Autodesk Inventor part; units mm, degrees
ref_plane "YZ Plane" through (0, 0, 0) normal (1, 0, 0) x (0, 1, 0)
ref_plane "XZ Plane" through (0, 0, 0) normal (0, 1, 0) x (-1, 0, 0)
ref_plane "XY Plane" through (0, 0, 0) normal (0, 0, 1) x (1, 0, 0)
sketch "Sketch1" plane through (0, 0, 0) normal (0, 1, 0) x (-1, 0, 0)
  line L0 (0, 0) -> (14, 0)
  line L1 (14, 0) -> (14, -8.75)
  line L2 (14, -8.75) -> (0, -8.75)
  line L3 (0, -8.75) -> (0, 0)
  line L4 (14, 0) -> (0, 0)
  line L5 (0, 0) -> (0, -8)
  line L6 (0, -8) -> (14, -8)
  line L7 (14, -8) -> (14, 0)
  line L8 (0, -8.75) -> (5.5, -8.75)
  line L9 (14, -8.75) -> (8.5, -8.75)
  line L10 (8.5, -8.75) -> (8.5, -4)
  line L11 (5.5, -8.75) -> (5.5, -4)
  line L12 (5.5, -8) -> (7, -8)
  line L13 (5.5, -8) -> (6.25, -8)
  line L14 (8.5, -8) -> (7, -8)
  line L15 (8.5, -8) -> (7.75, -8)
  line L16 (7.75, -8) -> (8.5, -8.75)
  line L17 (6.25, -8) -> (5.5, -8.75)
  dimension "d0" = 14
  dimension "d1" = 8.75
  dimension "d2" = 8
  dimension "d3" = 5.5
  dimension "d4" = 5.5
revolve "Revolution1" add sketch "Sketch1" angle 360 about axis through (0, 0, 0) along (-1, 0, 0) contours L0 L1 L6 L3 | L6 L11 L2 L3 | L1 L2 L10 L6 | L6 L17 L11 | L10 L16 L6
sketch "Sketch2" plane through (0, 0, 0) normal (1, 0, 0) x (0, 0, -1)
  circle A0 centre (0, 0) radius 1.5
  line L0 (-1.5, 0) -> (-1, 0)
  line L1 (-1, 0) -> (-1, 1.118)
  line L2 (-1, 0) -> (-1, -1.118)
  circle A1 centre (0, 0) radius 2.75
  dimension "d6" = 3
  dimension "d7" = 0.5
  dimension "d8" = 5.5
extrude "Extrusion1" cut sketch "Sketch2" against normal blind 10 contours A0 L2 L1
extrude "Extrusion2" cut sketch "Sketch2" against normal blind 0.6 contours L1 L0 A0 | A0 L0 L2 | A1
fillet "Fillet1" radius 20 1 edges at (0, 0, 2.75)
sketch "Sketch3" plane through (-14, 0, 0) normal (-1, 0, 0) x (0, 0, 1)
  circle A0 centre (0, 0) radius 8.75
  line L0 (0, -8.75) -> (0, -6.75)
  line L1 (0, 8.75) -> (0, 6.75)
  circle A1 centre (0, 0) radius 6.75
  dimension "d14" = 2
  dimension "d15" = 2
extrude "Extrusion3" cut sketch "Sketch3" against normal blind 1 contours A1
fillet "Fillet2" radius 0.5 1 edges at (-14, 0, -6.75)
sketch "Sketch4" plane through (-0.6, 0, 0) normal (1, 0, 0) x (0, 0, -1)
  circle A0 centre (0, 0) radius 2.75
  line L0 (-1, 1.118) -> (-1, -1.118)
  arc A1 (-1, -1.118) -> (-1, 1.118) centre (0, 0) ccw
  line L1 (1.5, 0) -> (1.6492, 0)
  line L2 (1.5, 0) -> (1.75, 0)
  circle A2 centre (0, 0) radius 1.75
  line L3 (-1, 1.118) -> (-1, -1.118)
  line L4 (-1, 0) -> (-1.25, 0)
  line L5 (-1.25, 0) -> (-1.25, 1.2247)
  line L6 (-1.25, 0) -> (-1.25, -1.2247)
  dimension "d19" = 0.25
  dimension "d20" = 0.25
extrude "Extrusion4" cut sketch "Sketch4" against normal blind 9.4 contours L0 L4 L5 A2 L2 L1 A1 | L0 A1 L1 L2 A2 L6 L4
sketch "Sketch5" plane through (-14, 0, 0) normal (-1, 0, 0) x (0, 0, 1)
  circle A0 centre (0, 0) radius 8.75
  circle A1 centre (0, 0) radius 7.25
  circle A2 centre (0, 0) radius 8.75
extrude "Extrusion5" add sketch "Sketch5" against normal blind 1 contours A0 | A1
sketch "Sketch6" plane through (-0.6, 0, 0) normal (1, 0, 0) x (0, 0, -1)
  arc A0 (-1.25, -1.2247) -> (-1.25, 1.2247) centre (0, 0) ccw
  line L0 (-1.25, -1.2247) -> (-1.25, 1.2247)
  circle A1 centre (0, 0) radius 2.75
  circle A2 centre (0, 0) radius 1.75
  line L1 (-1.25, -1.2247) -> (-1.25, 1.2247)
  line L2 (-1.25, 0) -> (-1, 0)
  line L3 (-1, 0) -> (-1, -1.4361)
  arc A3 (-1.25, -1.2247) -> (-1.25, 1.2247) centre (0, 0) ccw
  line L4 (-1, 0) -> (-1, 1.4361)
  dimension "d25" = 0.25
extrude "Extrusion6" add sketch "Sketch6" against normal blind 10 contours L0 L2 L3 A0 | L0 A0 L4 L2
properties part number "koło"
Could you check a few things on this model? Use its own coordinates, in mm. A direction names the side the tool comes from. Round coordinates to 2 decimals unless told otherwise and drop trailing zeros. Write each loop counter-clockwise with the first axis right and the second up, starting at its lowest first coordinate (ties: lowest second). Pieces come first, ordered by that corner, then holes. Notation, with made-up numbers: (-32, 40.25) - (26, 40.25) arc R16 ccw to (26, 50.25) - close; hole circle Ø7 at (51.5, 8.25). An arc over 180 degrees is marked (long way). Put each result on its own line as item: value. Start each with the question number.
(1) I want a section at A-A, the plane x = -10.5. Please give me the cut outline in (y, z).
(2) For faces 1 (the flat face through (-5, 0, 1)), 2 (the cylindrical face through (-2.712, -5.324, 6.944)), which set-ups out of +Z, -Z, +X, -X, +Y, -Y let a thin tool reach every point of the face, with its end or its side?
(3) Will these pins go through, and if not, where does the flat tip stop? pin 1 (6 mm diameter, centred on x = -6.5, z = -6, fed in from +Y) (3 decimals); pin 2 (1 mm diameter, centred on x = -2, y = 5, fed in from -Z); pin 3 (3 mm diameter, centred on y = 0, z = 0, fed in from +X).
(4) I need wall thicknesses on probe 1 along Y at (x, z) = (-7.25, 0); probe 2 along Y at (x, z) = (-4.5, 0); probe 3 along X at (y, z) = (6.5, -4.75). Which ranges of each line are inside material? Lowest first, please.
(5) I want a section at B-B, the plane x = -3. Please give me the cut outline in (y, z).
(6) Thinking about a two-plate mould opening in X: for faces 3 (the cylindrical face through (-5.23, -0.05, -1.75)), 4 (the cylindrical face through (-7.01, 7.81, 1.73)), 5 (the flat face through (-0.6, 0, 1.3)), which applies, released by +X, released by -X, zero draft, split by the parting line, or undercut?
Here are the results:
1. outline: circle Ø17.5 at (0, 0)
2. face 1: +X
2. face 2: +X, -X
3. pin 1: stops at y = 8.155
3. pin 2: stops at z = -7.5
3. pin 3: stops at x = -0.6
4. probe 1: y = -8 to -1.75, 1.75 to 8
4. probe 2: y = -8.75 to -1.75, 1.75 to 8.75
4. probe 3: x = -14 to -7.8, -6.2 to 0
5. outline: circle Ø17.5 at (0, 0); hole (-1.44, 1) arc R1.75 ccw (long way) to (1.44, 1) - close
6. face 3: zero draft
6. face 4: undercut
6. face 5: released by +X
